Design review of the part built by this model. Coordinates are the model's own, in mm. A direction names the side the tool comes from. Coordinates: 2 decimals unless noted, no trailing zeros. Loops run counter-clockwise (first coordinate to the right, second up) from the corner with the lowest first, then second, coordinate; pieces in that order, holes last. Notation, with made-up numbers: M -33,16 L 2,16 A12 cw 2,34 Z; hole C 42,16.25 d9. An arc over 180 degrees is marked long. Put each result on its own line as item: value. Start each with the question number.
(1) Take a section at A-A, the plane x = 53. Give the boundary of the cut face in (y, z).
(2) Take a section at C-C, the plane y = 1. Give the boundary of the cut face in (x, z), then the cut area to 3 significant figures.
(3) Take a section at D-D, the plane x = 27. Give the boundary of the cut face in (y, z), then the cut area to 3 significant figures.
(4) The part is to be moulded in two halves that separate along Y. For faces 4 (the cylindrical face through (9.231, -3.986, 11.897)), 5 (the cylindrical face through (83.12, 8.36, 1.48)), 6 (the flat face through (8, -3, 10)), say which applies: +Y half, -Y half, draft (parallel to the pull), parting line (faces both ways), or undercut.
(5) For faces 1 (the flat face through (0, -1, 8)), 2 (the flat face through (44, 6, 3)), 3 (the cylindrical face through (15.4, -1.5, 6.2)), list the 3-axis set-ups (+Z, -Z, +X, -X, +Y, -Y) from which the entire face can be reached by the end or side of a thin tool; tool diameter is ignored.
(6) Take a section at B-B, the plane z = 14. Give the boundary of the cut face in (x, y), then the cut area to 3 significant figures.
(7) Clearance check with flat-ended pins moving along their axes: pin 1 (5.5 mm diameter, centred on x = 83, y = 11.86, fed in from -Z); pin 2 (8.5 mm diameter, centred on x = 59, z = 12, fed in from +Y); pin 3 (7.5 mm diameter, centred on x = 36.5, y = 10, fed in from +Z); pin 4 (6 mm diameter, centred on x = 10.44, z = 10, fed in from +Y). State where each tip first meets the part, or that it passes through.
(8) For probe 1 along Z at (x, y) = (10.5, -1.75); probe 2 along Z at (x, y) = (80, -3.75); probe 3 along X at (y, z) = (-3.25, 12), list the stretches that pass through material, from the lowest coordinate up. Write a range as [from, to].
```python
from build123d import *

# Parameters (mm, degrees)
F0_W     = 90
F0_H     = 5
F1_DEPTH = 20
F2_R     = 6.25
F2_R_2   = 2.25
F3_DEPTH = 3
F4_DEPTH = 25
F5_DEPTH = 3


with BuildPart() as f1:
    # F0 (on Top) → F1 (new body)
    with BuildSketch(Plane.XY):
        with Locations((45, -2.5)):
            Rectangle(F0_W, F0_H)
    extrude(amount=F1_DEPTH)

    # F2 (on face) → F3 (cut)
    with BuildSketch(Plane(origin=(0, 0, 0), x_dir=(-1, 0, 0), z_dir=(0, 1, 0))):
        with Locations((-10.4403868318, 10)):
            Circle(F2_R)
        with Locations((-10.4403868318, 10)):
            Circle(F2_R_2, mode=Mode.SUBTRACT)
        with Locations((-80, 10)):
            Circle(F2_R)
        with Locations((-80, 10)):
            Circle(F2_R_2, mode=Mode.SUBTRACT)
    extrude(amount=-F3_DEPTH, mode=Mode.SUBTRACT)

    # F4 (cut): faces of the model
    f4_faces = [f1.faces().sort_by_distance(p)[0] for p in [
        (80, 0, 10),
        (10.4403868318, 0, 10),
    ]]
    extrude(f4_faces, amount=-F4_DEPTH, mode=Mode.SUBTRACT)

    # F0 (on Top) → F5 (join)
    with BuildSketch(Plane.XY):
        with BuildLine():
            Line((0, 13), (0, 0))
            Line((0, 0), (90, 0))
            Line((90, 0), (90, 11.8577008211))
            Line((90, 11.8577008211), (90, 14.8577008211))
            Line((90, 14.8577008211), (84.7905250274, 14.8650285595))
            ThreePointArc((84.7905250274, 14.8650285595), (82.9950768438, 8.3577042836), (81.2179423605, 14.8700538166))
            Line((81.2179423605, 14.8700538166), (74.7666283432, 14.8791283475))
            ThreePointArc((74.7666283432, 14.8791283475), (72.9950768438, 8.3577042836), (71.2418786162, 14.8840863219))
            Line((71.2418786162, 14.8840863219), (64.7422887653, 14.8932287584))
            ThreePointArc((64.7422887653, 14.8932287584), (62.9950768438, 8.3577042836), (61.2662577654, 14.8981182043))
            Line((61.2662577654, 14.8981182043), (54.7174874018, 14.9073298189))
            ThreePointArc((54.7174874018, 14.9073298189), (52.9950768438, 8.3577042836), (51.2910987002, 14.9121494371))
            Line((51.2910987002, 14.9121494371), (44.6922038807, 14.9214315577))
            ThreePointArc((44.6922038807, 14.9214315577), (42.99446615, 8.3577051959), (41.3174926972, 14.9267673202))
            Line((41.3174926972, 14.9267673202), (35.1435817461, 14.9377101925))
            ThreePointArc((35.1435817461, 14.9377101925), (33.9960120215, 10.7500035342), (32.8632943585, 14.9417518597))
            Line((32.8632943585, 14.9417518597), (28.1222277254, 14.9501551047))
            ThreePointArc((28.1222277254, 14.9501551047), (26.9960120215, 10.7500035342), (25.8846923606, 14.9541209966))
            Line((25.8846923606, 14.9541209966), (21.1003169088, 14.9626010038))
            ThreePointArc((21.1003169088, 14.9626010038), (19.9960120215, 10.7500035342), (18.9066471585, 14.9664891467))
            Line((18.9066471585, 14.9664891467), (14.0778151948, 14.9750479503))
            ThreePointArc((14.0778151948, 14.9750479503), (12.9960120215, 10.7500035342), (11.9291928539, 14.9788562494))
            Line((11.9291928539, 14.9788562494), (7.0546845996, 14.9874960114))
            ThreePointArc((7.0546845996, 14.9874960114), (5.9960120215, 10.7500035342), (4.9523674304, 14.9912222375))
            Line((4.9523674304, 14.9912222375), (0, 15))
            Line((0, 15), (0, 13))
        make_face()
    extrude(amount=F5_DEPTH)


solid = f1.part
```
Computed values:
1. outline: M -5,0 L 8.36,0 L 8.36,3 L 0,3 L 0,20 L -5,20 Z
2. outline: M 0,0 L 90,0 L 90,3 L 0,3 Z
2. area: 270 mm^2
3. outline: M -5,0 L 10.75,0 L 10.75,3 L 0,3 L 0,20 L -5,20 Z
3. area: 132 mm^2
4. face 4: draft
4. face 5: undercut
4. face 6: +Y half
5. face 1: +Z, -Z, -X, +Y, -Y
5. face 2: +Z, +X, -X, +Y
5. face 3: +Y
6. outline: M 0,-5 L 90,-5 L 90,0 L 84.8,0 L 84.8,-3 L 75.2,-3 L 75.2,0 L 15.24,0 L 15.24,-3 L 5.64,-3 L 5.64,0 L 0,0 Z
6. area: 392 mm^2
7. pin 1: passes through
7. pin 2: stops at y = 0
7. pin 3: stops at z = 3
7. pin 4: stops at y = -3
8. probe 1: z = [0, 3.75], [16.25, 20]
8. probe 2: z = [0, 7.75], [12.25, 20]
8. probe 3: x = [0, 9.41], [11.47, 78.97], [81.03, 90]
